Design review of the part built by this model. Coordinates are the model's own, in mm. Face numbers are marked on the shaded views. A direction names the side the tool comes from. Coordinates: 2 decimals unless noted, no trailing zeros. Loops run counter-clockwise (first coordinate to the right, second up) from the corner with the lowest first, then second, coordinate; pieces in that order, holes last. Notation, with made-up numbers: M 54,-35.5 L 74,-35.5 A4 cw 74,-28.5 Z; hole C 48,32.25 d8. An arc over 180 degrees is marked long. One line per item, written item: value.
```python
from build123d import *

# Parameters (mm, degrees)
SKETCH_1_R           = 270
EXTRUDE_1_DEPTH      = 13
SKETCH_2_R           = 150
SKETCH_2_R_2         = 120
EXTRUDE_2_DEPTH      = 400
CUT_EXTRUDE_1_DEPTH  = 220
EXTRUDE_3_DEPTH      = 60
SKETCH_27_W          = 165
SKETCH_27_H          = 165
EXTRUDE_14_DEPTH     = 30
SKETCH_51_R          = 122.82
CUT_EXTRUDE_20_DEPTH = 25
SKETCH_52_W          = 160
SKETCH_52_H          = 160
EXTRUDE_33_DEPTH     = 25
SKETCH_53_R          = 50
EXTRUDE_34_DEPTH     = 10


with BuildPart() as part:
    # 草图1 → 凸台-拉伸1 (new body)
    with BuildSketch(Plane.XY):
        with Locations(Location((0, 0, 0), (0, 0, 180))):
            Circle(SKETCH_1_R)
    extrude(amount=EXTRUDE_1_DEPTH)

    # 草图2 → 凸台-拉伸2 (add)
    with BuildSketch(Plane.XY):
        Circle(SKETCH_2_R)
        Circle(SKETCH_2_R_2, mode=Mode.SUBTRACT)
    extrude(amount=EXTRUDE_2_DEPTH)

    # 草图4 → 切除-拉伸1 (cut, symmetric)
    with BuildSketch(Plane(origin=(0, 0, 0), x_dir=(1, 0, 0), z_dir=(0, 1, 0))):
        with BuildLine():
            Line((-150, -113), (-150, -400))
            Line((-150, -400), (175.732568569, -400))
            ThreePointArc((175.732568569, -400), (150.72256284, -377.307091697), (131.640141985, -349.444398214))
            ThreePointArc((131.640141985, -349.444398214), (14.085885106, -203.509183955), (-150, -113))
        make_face()
    extrude(amount=CUT_EXTRUDE_1_DEPTH, both=True, mode=Mode.SUBTRACT)

    # 草图5 → 凸台-拉伸3 (add, symmetric)
    with BuildSketch(Plane(origin=(0, 0, 0), x_dir=(1, 0, 0), z_dir=(0, 1, 0))):
        with BuildLine():
            Line((131.640141985, -13), (235.929592589, -13))
            ThreePointArc((235.929592589, -13), (320.412645509, -107.525028653), (388.359858015, -214.555601786))
            ThreePointArc((388.359858015, -214.555601786), (327.444398214, -410.359858015), (131.640141985, -349.444398214))
            Line((131.640141985, -349.444398214), (131.640141985, -13))
        make_face()
    extrude(amount=EXTRUDE_3_DEPTH, both=True)

    # 草图27 → 凸台-拉伸14 (add)
    with BuildSketch(Plane.XY.offset(13)):
        Rectangle(SKETCH_27_W, SKETCH_27_H)
    extrude(amount=EXTRUDE_14_DEPTH)

    # 草图51 → 切除-拉伸20 (cut)
    with BuildSketch(Plane(origin=(0, 60, 0), x_dir=(1, 0, 0), z_dir=(0, 1, 0))):
        with Locations((260, -282)):
            Circle(SKETCH_51_R)
    extrude(amount=CUT_EXTRUDE_20_DEPTH, mode=Mode.SUBTRACT)

    # 草图52 → 凸台-拉伸33 (add)
    with BuildSketch(Plane(origin=(0, 60, 0), x_dir=(1, 0, 0), z_dir=(0, 1, 0))):
        with Locations((260, -282)):
            Rectangle(SKETCH_52_W, SKETCH_52_H)
    extrude(amount=EXTRUDE_33_DEPTH)

    # 草图53 → 凸台-拉伸34 (add)
    with BuildSketch(Plane(origin=(0, -60, 0), x_dir=(-1, 0, 0), z_dir=(0, -1, 0))):
        with Locations(Location((-260, -282, 0), (0, 0, 270))):
            Circle(SKETCH_53_R)
    extrude(amount=EXTRUDE_34_DEPTH)


solid = part.part
```
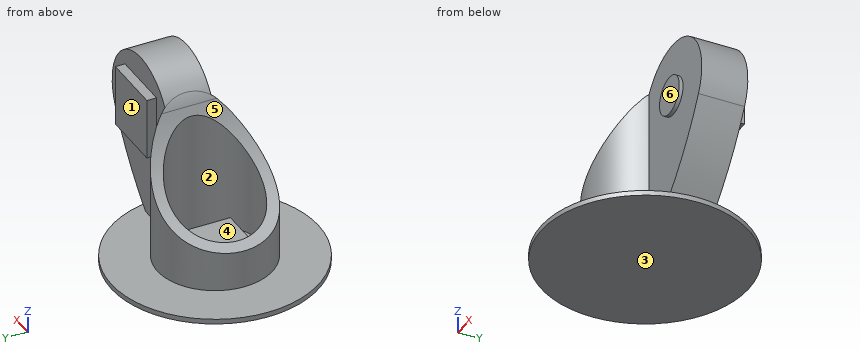
(1) We need section A-A on x = 260. State the section outline as (y, z) points, then the cut area to 3 significant figures.
Reply:
outline: M -72.8,0 L 72.8,0 L 72.8,13 L -72.8,13 Z; M -70,232 L -60,232 L -60,36.88 L 60,36.88 L 60,202 L 85,202 L 85,362 L 60,362 L 60,427 L -60,427 L -60,332 L -70,332 Z
area: 53,700 mm2
(2) Mouldability with a two-part tool opening along X and no side actions: class the marked faces 4, 5 and 6 as released by +X, released by -X, zero draft, split by the parting line, or undercut.
Reply:
face 4: undercut
face 5: released by -X
face 6: zero draft
(3) We need section B-B on z = 121. State the section outline as (x, y) points.
Reply:
outline: M -127.01,-79.81 A150 ccw 137.48,-60 L 330.38,-60 L 330.38,60 L 137.48,60 A150 ccw -127.01,79.81 Z; hole C 0,0 d240
(4) We need section D-D on z = 340.5. State the section outline as (x, y) points.
Reply:
outline: M 126.82,-80.1 A150 ccw 137.48,-60 L 392.68,-60 L 392.68,60 L 340,60 L 340,85 L 180,85 L 180,60 L 137.48,60 A150 ccw 126.82,80.1 Z
(5) Tool access review of the marked faces 1, 2 and 3: name each direction out of +Z, -Z, +X, -X, +Y, -Y from which nothing blocks a thin tool from reaching the whole face with its end or side.
Reply:
face 1: +Z, +X, +Y
face 2: +Z
face 3: -Z, +X, -X, +Y, -Y
(6) Insertion check: pin 1 (9 mm diameter, centred on y = -31.5, z = 33, fed in from -X); pin 2 (7.5 mm diameter, centred on x = 239.5, y = 75, fed in from +Z); pin 3 (9 mm diameter, centred on x = 22.5, z = 21.5, fed in from +Y). Each pin has a flat end and moves straight along its axis. Give the tip position at first contact, or say it passes through.
Reply:
pin 1: stops at x = -147.55
pin 2: stops at z = 362
pin 3: stops at y = 148.92
(7) To check wall thickness, follow line 1 along Y through (x, z) = (0, 103); line 2 along Z through (x, y) = (-137, -106.5); line 3 along Y through (x, z) = (333.5, 143.5). State the ranges of each line that lie inside material, in increasing order. Write a range as [from, to].
Reply:
line 1: y = [-150, -120], [120, 150]
line 2: z = [0, 13]
line 3: y = [-60, 60]
(8) We need section C-C on y = 0. State the section outline as (x, z) points, then the cut area to 3 significant figures.
Reply:
outline: M -270,0 L 270,0 L 270,13 L 235.93,13 A775.24 ccw 388.36,214.56 A145 ccw 131.64,349.44 A485.24 cw 120,328.56 L 120,13 L 82.5,13 L 82.5,43 L -82.5,43 L -82.5,13 L -120,13 L -120,123.7 A485.24 cw -150,113 L -150,13 L -270,13 Z
area: 107,000 mm2
